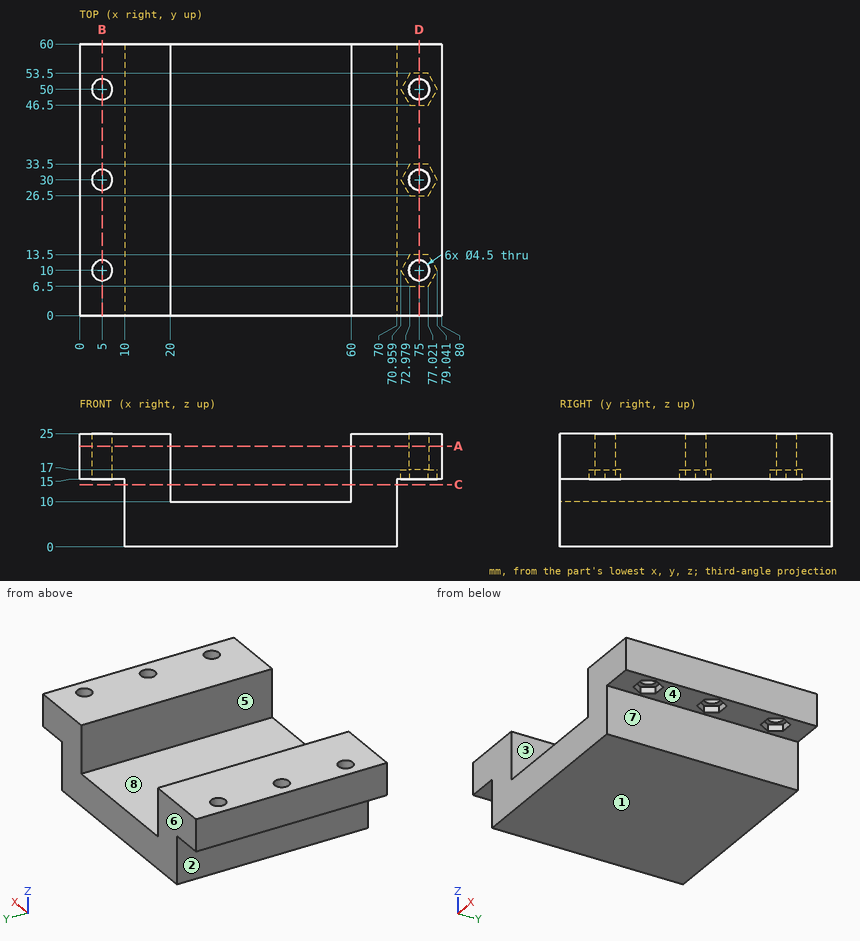
Job drawing, mm, ordinate dimensions from the low corner. One solid piece. A direction names the side the tool comes from. Give positions to 0.01 mm unless a question says otherwise; leave off trailing zeros. Loops run counter-clockwise (first coordinate to the right, second up) from the corner with the lowest first, then second, coordinate; pieces in that order, holes last. Notation, with made-up numbers: M 82,70.5 L 118,70.5 A15 cw 118,95.5 Z; hole C -31.75,48.5 d2. An arc over 180 degrees is marked long. Put each result on its own line as item: value. Start each with the question number.
1) Pull direction X, two halves, no side cores. Call the marked faces 5, 6, 7 and 8: +X half, -X half, draft (parallel to the pull), parting line (faces both ways), or undercut.
2) Saw through at D-D (x = 75). List the corners of the cut face in (y, z), then the cut area to 3 significant figures.
3) Probe probe 1 along Y at (x, z) = (75, 19); probe 2 along X at (y, z) = (21.5, 16.5); probe 3 along X at (y, z) = (55, 12). List the from-to ranges inside material, lowest first.
4) Saw through at C-C (z = 13.75). List the corners of the cut face in (x, y).
5) Flat gauge pins, fed straight in: pin 1 (1.5 mm diameter, centred on y = 23.5, z = 3, fed in from +X); pin 2 (6 mm diameter, centred on x = 75, y = 10, fed in from -Z); pin 3 (7.5 mm diameter, centred on x = 77, y = 8.5, fed in from -Z). Where does each tip first touch, or does it go through?
6) 3-axis set-ups, long thin cutter, end or side, ignore diameter. For the marked faces 1, 2, 3 and 4: which of +Z, -Z, +X, -X, +Y, -Y reach the whole face in a straight line?
7) Saw through at A-A (z = 22.25). List the corners of the cut face in (x, y), then the cut area to 3 significant figures.
8) Saw through at B-B (x = 5). List the corners of the cut face in (y, z), then the cut area to 3 significant figures.
Numbers:
1. face 5: undercut
1. face 6: draft
1. face 7: +X half
1. face 8: undercut
2. outline: M 0,15 L 6.5,15 L 6.5,17 L 7.75,17 L 7.75,25 L 0,25 Z; M 12.25,17 L 13.5,17 L 13.5,15 L 26.5,15 L 26.5,17 L 27.75,17 L 27.75,25 L 12.25,25 Z; M 32.25,17 L 33.5,17 L 33.5,15 L 46.5,15 L 46.5,17 L 47.75,17 L 47.75,25 L 32.25,25 Z; M 52.25,17 L 53.5,17 L 53.5,15 L 60,15 L 60,25 L 52.25,25 Z
2. area: 450 mm^2
3. probe 1: 0 to 7.75, 12.25 to 27.75, 32.25 to 47.75, 52.25 to 60
3. probe 2: 0 to 20, 60 to 80
3. probe 3: 10 to 20, 60 to 70
4. outline: M 10,0 L 20,0 L 20,60 L 10,60 Z; M 60,0 L 70,0 L 70,60 L 60,60 Z
5. pin 1: x = 70
5. pin 2: z = 17
5. pin 3: z = 15
6. face 1: -Z, +X, -X, +Y, -Y
6. face 2: -Z, -X, +Y, -Y
6. face 3: +Z, +Y, -Y
6. face 4: -Z, +X, +Y, -Y
7. outline: M 0,0 L 20,0 L 20,60 L 0,60 Z; M 60,0 L 80,0 L 80,60 L 60,60 Z; hole C 5,10 d4.5; hole C 5,30 d4.5; hole C 5,50 d4.5; hole C 75,10 d4.5; hole C 75,30 d4.5; hole C 75,50 d4.5
7. area: 2,300 mm^2
8. outline: M 0,15 L 7.75,15 L 7.75,25 L 0,25 Z; M 12.25,15 L 27.75,15 L 27.75,25 L 12.25,25 Z; M 32.25,15 L 47.75,15 L 47.75,25 L 32.25,25 Z; M 52.25,15 L 60,15 L 60,25 L 52.25,25 Z
8. area: 465 mm^2
